Can you work these out from the model? Positions are in its coordinate system, mm. Face numbers are marked on the shaded views. A direction names the side the tool comes from. Give positions to 0.01 mm unless a question says otherwise; leave off trailing zeros. Write each loop counter-clockwise with the first axis right and the second up, starting at its lowest first coordinate (ties: lowest second). Pieces come first, ordered by that corner, then holes.
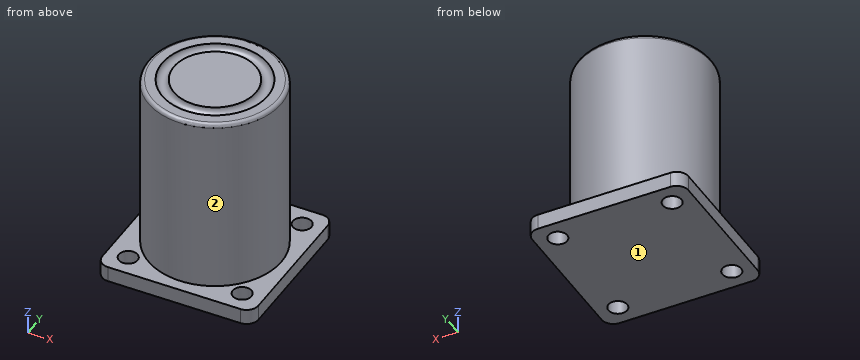
```python
from build123d import *

# Parameters (mm, degrees)
TORUS_R           = 1.5
CYLINDER004_R     = 17
CYLINDER004_DEPTH = 50
FILLET001_R       = 1
CYLINDER002_R     = 2.4
CYLINDER002_DEPTH = 10
CYLINDER001_R     = 2.4
CYLINDER001_DEPTH = 10
CYLINDER_R        = 2.4
CYLINDER_DEPTH    = 10
CYLINDER003_R     = 2.4
CYLINDER003_DEPTH = 10
BOX_W             = 40
BOX_H             = 40
BOX_DEPTH         = 4
FILLET_R          = 3


with BuildPart() as torus:
    # Torus → Torus (revolve)
    with BuildSketch(Plane(origin=(20, 20, 50), x_dir=(1, 0, 0), z_dir=(0, -1, 0))):
        with Locations((12, 0)):
            Circle(TORUS_R)
    revolve(axis=Axis((20, 20, 50), (0, 0, 1)))


with BuildPart() as fillet001:
    # Cylinder004 → Cylinder004 (new body)
    with BuildSketch(Plane(origin=(20, 20, 0), x_dir=(1, 0, 0), z_dir=(0, 0, 1))):
        Circle(CYLINDER004_R)
    extrude(amount=CYLINDER004_DEPTH)

    # Fillet001
    fillet001_edges = [fillet001.edges().sort_by_distance(p)[0] for p in [
        (3, 20, 50),
    ]]
    fillet(fillet001_edges, radius=FILLET001_R)


with BuildPart() as cilindre002:
    # Cylinder002 → Cylinder002 (new body)
    with BuildSketch(Plane(origin=(5.4, 5.4, 0), x_dir=(1, 0, 0), z_dir=(0, 0, 1))):
        Circle(CYLINDER002_R)
    extrude(amount=CYLINDER002_DEPTH)


with BuildPart() as cilindre001:
    # Cylinder001 → Cylinder001 (new body)
    with BuildSketch(Plane(origin=(5.4, 34.6, 0), x_dir=(1, 0, 0), z_dir=(0, 0, 1))):
        Circle(CYLINDER001_R)
    extrude(amount=CYLINDER001_DEPTH)


with BuildPart() as fusion:
    # Cylinder → Cylinder (new body)
    with BuildSketch(Plane(origin=(34.6, 34.8, 0), x_dir=(1, 0, 0), z_dir=(0, 0, 1))):
        Circle(CYLINDER_R)
    extrude(amount=CYLINDER_DEPTH)

    # Fusion: union Cilindre001
    add(cilindre001.part)


with BuildPart() as fusion001:
    # Cylinder003 → Cylinder003 (new body)
    with BuildSketch(Plane(origin=(34.6, 5.4, 0), x_dir=(1, 0, 0), z_dir=(0, 0, 1))):
        Circle(CYLINDER003_R)
    extrude(amount=CYLINDER003_DEPTH)

    # Fusion001: union Fusion
    add(fusion.part)


with BuildPart() as cut002:
    # Box → Box (new body)
    with BuildSketch(Plane.XY):
        with Locations((20, 20)):
            Rectangle(BOX_W, BOX_H)
    extrude(amount=BOX_DEPTH)

    # Cut: cut Fusion001
    add(fusion001.part, mode=Mode.SUBTRACT)

    # Cut001: cut Cilindre002
    add(cilindre002.part, mode=Mode.SUBTRACT)

    # Fillet
    fillet_edges = [cut002.edges().sort_by_distance(p)[0] for p in [
        (0, 0, 2),
        (0, 40, 2),
        (40, 0, 2),
        (40, 40, 2),
    ]]
    fillet(fillet_edges, radius=FILLET_R)

    # Fusion002: union Fillet001
    add(fillet001.part)

    # Cut002: cut Torus
    add(torus.part, mode=Mode.SUBTRACT)


solid = cut002.part
```
1) For the marked faces 1 and 2, which set-ups out of +Z, -Z, +X, -X, +Y, -Y let a thin tool reach every point of the face, with its end or its side?
Values follow:
face 1: -Z, +X, -X, +Y, -Y
face 2: +Z
2) Suppose I cut it at A-A on z = 45.5. Write out the boundary of the cut face in (x, y).
Values follow:
outline: circle Ø34 at (20, 20)
3) For pin 1 Ø1 at (y, z) = (4.5, 17) entering from +X; pin 2 Ø8 at (x, z) = (32, 40.5) entering from -Y; pin 3 Ø3 at (y, z) = (28, 20.5) entering from -X, each with a flat end and sliding along its axis, tell me the tip position at first contact or that it passes through.
Values follow:
pin 1: stops at x = 28
pin 2: stops at y = 5
pin 3: stops at x = 4.29
4) Please list where these lines run through material, in increasing order: L1, parallel to Y at x = 34.6, z = 1.15; L2, parallel to X at y = 5.4, z = 0.9.
Values follow:
L1: y = 0 to 3, 7.8 to 32.4, 37.2 to 40
L2: x = 0 to 3, 7.8 to 32.2, 37 to 40
5) Suppose I cut it at B-B on y = 5.4. State how many separate pieces and enclosed holes the cut face has, plus the area to 3 significant figures.
Values follow:
separate pieces: 3
enclosed holes: 0
area: 922 mm2
